Could you check a few things on this model? Use its own coordinates, in mm. A direction names the side the tool comes from. Give positions to 0.01 mm unless a question says otherwise; leave off trailing zeros. Order: outer loops, then holes, each group sorted by start corner. A loop starts at its lowest first (then second) coordinate and runs counter-clockwise, first axis right, second up.
(1) Will these pins go through, and if not, where does the flat tip stop? pin 1 (1.5 mm diameter, centred on y = -2, z = 37, fed in from -X); pin 2 (2.5 mm diameter, centred on x = 2, z = 17.5, fed in from +Y); pin 3 (1 mm diameter, centred on y = 1, z = 14, fed in from +X).
(2) If we mould it in two halves opening along X, with no side actions, what happens to faces 1 (the cylindrical face through (9.699, 9.715, 25.35)), 2 (the flat face through (4.19, -5.25, 24.65)), 3 (the flat face through (-3.901, -2, 25))? For each: released by +X, released by -X, zero draft, split by the parting line, or undercut.
(3) Imagine slicing it at B-B, the plane y = 1.25. Write out the boundary of the cut face in (x, z), then the cut area to 3 significant figures.
(4) Imagine slicing it at A-A, the plane y = -7.25. Write out the boundary of the cut face in (x, z), then the cut area to 3 significant figures.
(5) On a 3-axis mill with a long thin cutter (end or side, diameter ignored), from which of +Z, -Z, +X, -X, +Y, -Y can I reach the whole of each face in a straight line? I mean faces 4 (the flat face through (9.3, -3.7, 24.6)), 5 (the flat face through (-9.3, 3.7, 24.6)), 6 (the flat face through (2, -3.901, 25)), 7 (the flat face through (-5.499, 7, 25)). Say none if no direction works.
(6) If I drill on probe 1 along X at (y, z) = (7.75, 11.5); probe 2 along X at (y, z) = (-4, 13.5); probe 3 along Y at (x, z) = (5, 42), over which ranges is the centre line in solid material (lowest first)?
from build123d import *

# Parameters (mm, degrees)
SKETCH_1_R      = 2.1
EXTRUDE_1_DEPTH = 50
FILLET_1_R      = 1
FILLET_2_R      = 0.3


with BuildPart() as part:
    # Эскиз1 → Бобышка-Вытянуть1 (new body)
    with BuildSketch(Plane.XY):
        Polygon((-10, 10), (-4.4, 10), (-2.6, 8.2), (-5.499339828, 8.2), (-5.499339828, 6.56), (-2.84, 3.900660172), (-0.5, 3.900660172), (0, 3.400660172), (0.5, 3.900660172), (2.84, 3.900660172), (5.499339828, 6.56), (5.499339828, 8.2), (2.6, 8.2), (4.4, 10), (10, 10), (10, 4.4), (8.2, 2.6), (8.2, 5.499339828), (6.56, 5.499339828), (3.900660172, 2.84), (3.900660172, 0.5), (3.400660172, 0), (3.900660172, -0.5), (3.900660172, -2.84), (6.56, -5.499339828), (8.2, -5.499339828), (8.2, -2.6), (10, -4.4), (10, -10), (4.4, -10), (2.6, -8.2), (5.499339828, -8.2), (5.499339828, -6.56), (2.84, -3.900660172), (0.5, -3.900660172), (0, -3.400660172), (-0.5, -3.900660172), (-2.84, -3.900660172), (-5.499339828, -6.56), (-5.499339828, -8.2), (-2.6, -8.2), (-4.4, -10), (-10, -10), (-10, -4.4), (-8.2, -2.6), (-8.2, -5.499339828), (-6.56, -5.499339828), (-3.900660172, -2.84), (-3.900660172, -0.5), (-3.400660172, 0), (-3.900660172, 0.5), (-3.900660172, 2.84), (-6.56, 5.499339828), (-8.2, 5.499339828), (-8.2, 2.6), (-10, 4.4), align=None)
        Circle(SKETCH_1_R, mode=Mode.SUBTRACT)
    extrude(amount=EXTRUDE_1_DEPTH)

    # Скругление1
    fillet_1_edges = [part.edges().sort_by_distance(p)[0] for p in [
        (-10, 10, 25),
        (10, 10, 25),
        (10, -10, 25),
        (-10, -10, 25),
    ]]
    fillet(fillet_1_edges, radius=FILLET_1_R)

    # Скругление2
    fillet_2_edges = [part.edges().sort_by_distance(p)[0] for p in [
        (-4.4, 10, 25),
        (-2.6, 8.2, 25),
        (-5.499339828, 8.2, 25),
        (-5.499339828, 6.56, 25),
        (-2.84, 3.900660172, 25),
        (-0.5, 3.900660172, 25),
        (0.5, 3.900660172, 25),
        (2.84, 3.900660172, 25),
        (5.499339828, 6.56, 25),
        (5.499339828, 8.2, 25),
        (2.6, 8.2, 25),
        (4.4, 10, 25),
        (10, 4.4, 25),
        (8.2, 2.6, 25),
        (8.2, 5.499339828, 25),
        (6.56, 5.499339828, 25),
        (3.900660172, 2.84, 25),
        (3.900660172, 0.5, 25),
        (3.900660172, -0.5, 25),
        (3.900660172, -2.84, 25),
        (6.56, -5.499339828, 25),
        (8.2, -5.499339828, 25),
        (8.2, -2.6, 25),
        (10, -4.4, 25),
        (4.4, -10, 25),
        (2.6, -8.2, 25),
        (5.499339828, -8.2, 25),
        (5.499339828, -6.56, 25),
        (2.84, -3.900660172, 25),
        (0.5, -3.900660172, 25),
        (-0.5, -3.900660172, 25),
        (-2.84, -3.900660172, 25),
        (-5.499339828, -6.56, 25),
        (-5.499339828, -8.2, 25),
        (-2.6, -8.2, 25),
        (-4.4, -10, 25),
        (-10, -4.4, 25),
        (-8.2, -2.6, 25),
        (-8.2, -5.499339828, 25),
        (-6.56, -5.499339828, 25),
        (-3.900660172, -2.84, 25),
        (-3.900660172, -0.5, 25),
        (-3.900660172, 0.5, 25),
        (-3.900660172, 2.84, 25),
        (-6.56, 5.499339828, 25),
        (-8.2, 5.499339828, 25),
        (-8.2, 2.6, 25),
    ]]
    fillet(fillet_2_edges, radius=FILLET_2_R)


solid = part.part
Answer block:
1. pin 1: stops at x = -3.9
1. pin 2: stops at y = 8.85
1. pin 3: stops at x = 3.9
2. face 1: released by +X
2. face 2: undercut
2. face 3: released by -X
3. outline: (-3.9, 0) - (-1.69, 0) - (-1.69, 50) - (-3.9, 50) - close; (1.69, 0) - (3.9, 0) - (3.9, 50) - (1.69, 50) - close
3. area: 221 mm2
4. outline: (-10, 0) - (-5.5, 0) - (-5.5, 50) - (-10, 50) - close; (5.5, 0) - (10, 0) - (10, 50) - (5.5, 50) - close
4. area: 450 mm2
5. face 4: +Z, -Z, +X
5. face 5: +Z, -Z, -X
5. face 6: +Z, -Z, -Y
5. face 7: +Z, -Z
6. probe 1: x = -10 to -5.5, 5.5 to 10
6. probe 2: x = -9.6 to -8.2, -5.06 to -2.94, 2.94 to 5.06, 8.2 to 9.6
6. probe 3: y = -10 to -8.2, -6.06 to -3.94, 3.94 to 6.06, 8.2 to 10
